The figure shows three views and two pictorial views of one solid part (mm, origin at its lowest corner). Answer the questions. A direction names the side the tool comes from. Coordinates: 2 decimals unless noted, no trailing zeros. Order: outer loops, then holes, each group sorted by start corner. A loop starts at its lowest first (then second) coordinate and runs counter-clockwise, first axis right, second up. Notation, with made-up numbers: (89, 30) -> (100, 30) arc R20 ccw to (100, 43) -> close; hole circle Ø6 at (31, 37.5). An arc over 180 degrees is marked (long way). Return JSON: item names as keys, results as strings.
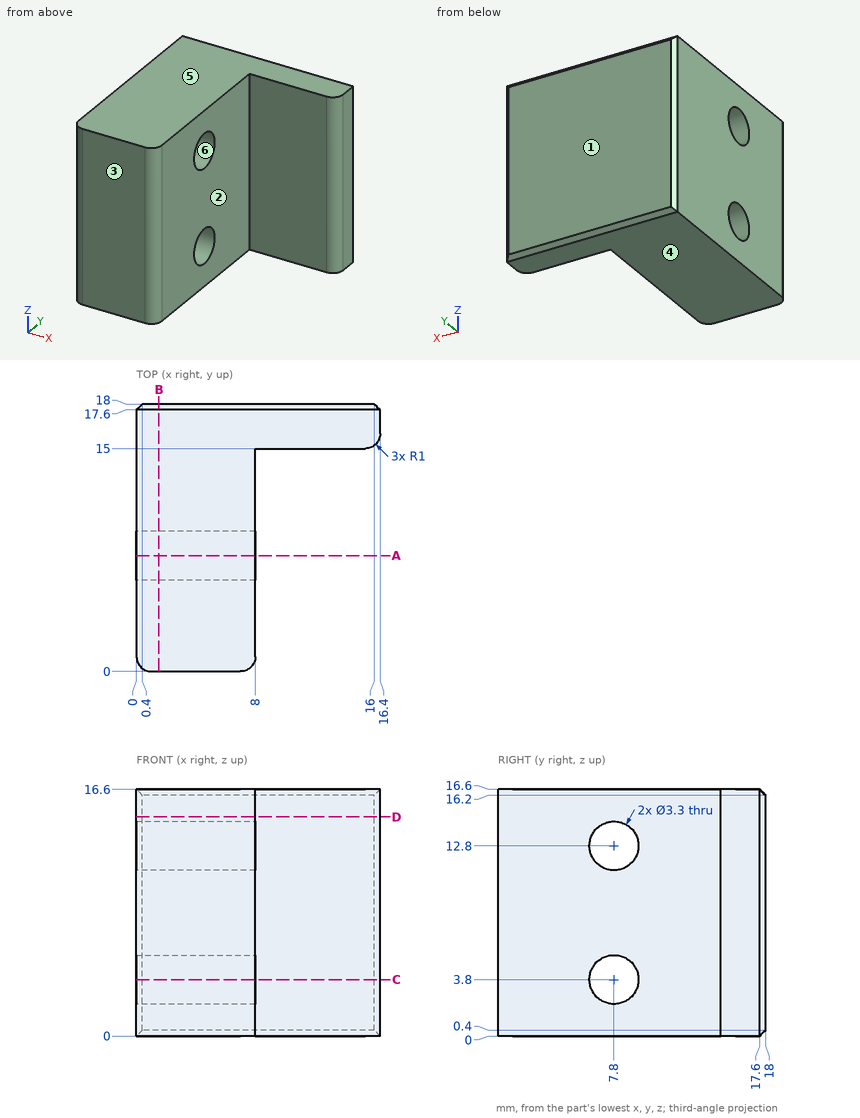
1. The part is cut by section D-D on z = 14.75. Give the vertices of the cut face in (x, y), and give its area (3 significant figures).
Answer block:
{"outline": "(0, 1) arc R1 ccw to (1, 0) -> (7, 0) arc R1 ccw to (8, 1) -> (8, 15) -> (15.4, 15) arc R1 ccw to (16.4, 16) -> (16.4, 17.6) -> (16, 18) -> (0.4, 18) -> (0, 17.6) -> close", "area": "168 mm2"}
2. For the marked faces 1 and 2, determine the directions among +Z, -Z, +X, -X, +Y, -Y from which every point of the face is accessible in a straight line to the end or side of a thin tool.
Answer block:
{"face 1": "+Z, -Z, +X, -X, +Y", "face 2": "+Z, -Z, +X, -Y"}
3. Consider line 1 (Y direction, x = 4.5, z = 3.8); line 2 (Y direction, x = 11.25, z = 3.25); line 3 (X direction, y = 7, z = 7.25). Determine where each line is inside the solid, lowest interval first. Write a range as from..to.
Answer block:
{"line 1": "y = 0..6.15, 9.45..18", "line 2": "y = 15..18", "line 3": "x = 0..8"}
4. The part is cut by section C-C on z = 3.8. Give the vertices of the cut face in (x, y).
Answer block:
{"outline": "(0, 1) arc R1 ccw to (1, 0) -> (7, 0) arc R1 ccw to (8, 1) -> (8, 6.15) -> (0, 6.15) -> close; (0, 9.45) -> (8, 9.45) -> (8, 15) -> (15.4, 15) arc R1 ccw to (16.4, 16) -> (16.4, 17.6) -> (16, 18) -> (0.4, 18) -> (0, 17.6) -> close"}
5. The part is cut by section A-A on y = 7.8. Give the vertices of the cut face in (x, z).
Answer block:
{"outline": "(0, 0) -> (8, 0) -> (8, 2.15) -> (0, 2.15) -> close; (0, 5.45) -> (8, 5.45) -> (8, 11.15) -> (0, 11.15) -> close; (0, 14.45) -> (8, 14.45) -> (8, 16.6) -> (0, 16.6) -> close"}
6. Determine the mould class of the marked faces 3, 4, 5 and 6 for opening direction Z: pulls with the +Z half, pulls with the -Z half, needs draft (parallel to the pull), parting line crosses it, or undercut.
Answer block:
{"face 3": "needs draft", "face 4": "pulls with the -Z half", "face 5": "pulls with the +Z half", "face 6": "undercut"}
7. The part is cut by section B-B on x = 1.5. Give the vertices of the cut face in (y, z), and give its area (3 significant figures).
Answer block:
{"outline": "(0, 0) -> (17.6, 0) -> (18, 0.4) -> (18, 16.2) -> (17.6, 16.6) -> (0, 16.6) -> close; hole circle Ø3.3 at (7.8, 3.8); hole circle Ø3.3 at (7.8, 12.8)", "area": "282 mm2"}
